from build123d import *

# Parameters (mm, degrees)
F0_R     = 3.5
F0_R_2   = 1.5
F1_DEPTH = 3
F2_R     = 3.5
F3_DEPTH = 1
F4_R     = 0.99999


# Not quite as in the source:
# - a fillet or chamfer is up to 0.001 mm smaller than in the source, because OpenCascade refuses the exact size


with BuildPart() as f1:
    # F0 (on Top) → F1 (new body)
    with BuildSketch(Plane.XY):
        Circle(F0_R)
        Circle(F0_R_2, mode=Mode.SUBTRACT)
    extrude(amount=F1_DEPTH)

    # F2 (on Top) → F3 (join)
    with BuildSketch(Plane.XY):
        Circle(F2_R)
    extrude(amount=-F3_DEPTH)

    # F4 (radius 1 in the source; OpenCascade refuses exactly that, so slightly less here)
    f4_edges = [f1.edges().sort_by_distance(p)[0] for p in [
        (-3.5, 0, -1),
    ]]
    fillet(f4_edges, radius=F4_R)


solid = f1.part
Design review of the part built by this model. Coordinates are the model's own, in mm. A direction names the side the tool comes from. Give positions to 0.01 mm unless a question says otherwise; leave off trailing zeros. Loops run counter-clockwise (first coordinate to the right, second up) from the corner with the lowest first, then second, coordinate; pieces in that order, holes last. Notation, with made-up numbers: (-2, 2) - (45, 2) arc R20 ccw to (45, 27) - close; hole circle Ø7 at (-1.75, 18). An arc over 180 degrees is marked (long way). Write item = value, one per line.
1) Take a section at C-C on z = 0.6. State the section outline as (x, y) points, and give its area (3 significant figures).
Result sheet:
outline = circle Ø7 at (0, 0); hole circle Ø3 at (0, 0)
area = 31.4 mm2
2) Clearance check with flat-ended pins moving along their axes: pin 1 Ø2 at (y, z) = (-1.5, 1.5) entering from -X; pin 2 Ø1.5 at (x, y) = (0, -0.5) entering from +Z. State where each tip first meets the part, or that it passes through.
Result sheet:
pin_1 = -3.46
pin_2 = 0
3) Take a section at A-A on y = 0. State the section outline as (x, z) points.
Result sheet:
outline = (-3.5, 0) arc R1 ccw to (-2.5, -1) - (2.5, -1) arc R1 ccw to (3.5, 0) - (3.5, 3) - (1.5, 3) - (1.5, 0) - (-1.5, 0) - (-1.5, 3) - (-3.5, 3) - close
4) To check wall thickness, follow line 1 (Y direction, x = 0, z = 1.6); line 2 (Z direction, x = -1, y = 0); line 3 (X direction, y = -0.5, z = 2). State the ranges of each line that lie inside material, in increasing order.
Result sheet:
line_1 = -3.5 to -1.5, 1.5 to 3.5
line_2 = -1 to 0
line_3 = -3.46 to -1.41, 1.41 to 3.46
5) Tool access review of faces 1 (the face through (0, 0, -1)), 2 (the face through (-1.5, 0.07, 1.48)): name each direction out of +Z, -Z, +X, -X, +Y, -Y from which nothing blocks a thin tool from reaching the whole face with its end or side.
Result sheet:
face_1 = -Z, +X, -X, +Y, -Y
face_2 = +Z
6) Draft analysis for pull direction Y (two halves, no side actions). For faces 3 (the face through (3.233, -1.341, 1.521)), 4 (the face through (0, 0, 0)), 5 (the face through (0, -2, 3)), state which applies: +Y half, -Y half, draft (parallel to the pull), parting line (faces both ways), or undercut.
Result sheet:
face_3 = parting line
face_4 = undercut
face_5 = draft
